The figure shows three views and two pictorial views of one solid part (mm, origin at its lowest corner). Answer the questions. A direction names the side the tool comes from. Coordinates: 2 decimals unless noted, no trailing zeros. Order: outer loops, then holes, each group sorted by start corner. A loop starts at its lowest first (then second) coordinate and runs counter-clockwise, first axis right, second up. Notation, with made-up numbers: (-16, -1) -> (4, -1) arc R22 cw to (4, 37) -> close; hole circle Ø9 at (6.25, 38). An arc over 180 degrees is marked (long way). Return JSON: item names as keys, results as strings.
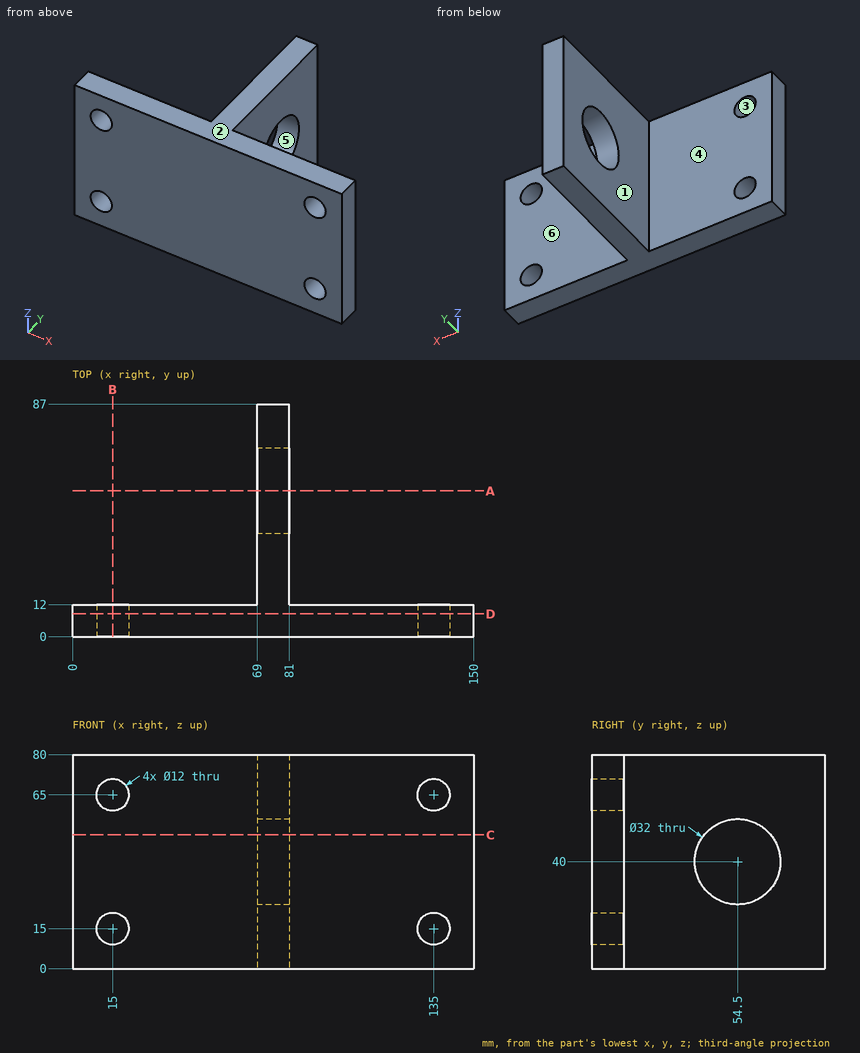
1. Consider line 1 (X direction, y = 5.25, z = 15); line 2 (Y direction, x = 101.5, z = 65); line 3 (X direction, y = 81, z = 33). Determine where each line is inside the solid, lowest interval first. Write a range as from..to.
Answer block:
{"line 1": "x = 0..9, 21..129, 141..150", "line 2": "y = 0..12", "line 3": "x = 69..81"}
2. The part is cut by section D-D on y = 8.5. Give the vertices of the cut face in (x, z), and give its area (3 significant figures).
Answer block:
{"outline": "(0, 0) -> (150, 0) -> (150, 80) -> (0, 80) -> close; hole circle Ø12 at (15, 15); hole circle Ø12 at (15, 65); hole circle Ø12 at (135, 15); hole circle Ø12 at (135, 65)", "area": "11,500 mm2"}
3. For the marked faces 4, 5 and 6, determine the directions among +Z, -Z, +X, -X, +Y, -Y from which every point of the face is accessible in a straight line to the end or side of a thin tool.
Answer block:
{"face 4": "+Z, -Z, -X, +Y", "face 5": "+X, -X", "face 6": "+Z, -Z, +X, +Y"}
4. Each of these flat-tipped pins is pushed along its axis until it touches: pin 1 Ø2 at (y, z) = (48, 63) entering from -X; pin 2 Ø20.5 at (x, z) = (42, 26.5) entering from +Y; pin 3 Ø7 at (x, z) = (135, 65) entering from +Y (3 decimals). Where does it stop, or does it pass through?
Answer block:
{"pin 1": "stops at x = 69", "pin 2": "stops at y = 12", "pin 3": "passes through"}
5. The part is cut by section B-B on x = 15. Give the vertices of the cut face in (y, z), and give its area (3 significant figures).
Answer block:
{"outline": "(0, 0) -> (12, 0) -> (12, 9) -> (0, 9) -> close; (0, 21) -> (12, 21) -> (12, 59) -> (0, 59) -> close; (0, 71) -> (12, 71) -> (12, 80) -> (0, 80) -> close", "area": "672 mm2"}
6. The part is cut by section A-A on y = 54.5. Give the vertices of the cut face in (x, z), and give its area (3 significant figures).
Answer block:
{"outline": "(69, 0) -> (81, 0) -> (81, 24) -> (69, 24) -> close; (69, 56) -> (81, 56) -> (81, 80) -> (69, 80) -> close", "area": "576 mm2"}
7. Determine the mould class of the marked faces 1, 2 and 3 for opening direction X: pulls with the +X half, pulls with the -X half, needs draft (parallel to the pull), parting line crosses it, or undercut.
Answer block:
{"face 1": "pulls with the -X half", "face 2": "needs draft", "face 3": "undercut"}
8. The part is cut by section C-C on z = 50. Give the vertices of the cut face in (x, y).
Answer block:
{"outline": "(0, 0) -> (150, 0) -> (150, 12) -> (81, 12) -> (81, 42.01) -> (69, 42.01) -> (69, 12) -> (0, 12) -> close; (69, 66.99) -> (81, 66.99) -> (81, 87) -> (69, 87) -> close"}
